from build123d import *

# Parameters (mm, degrees)
ESBO_O1_R           = 30
ESBO_O1_R_2         = 25
BOSS_EXTRUDE1_DEPTH = 1.57
BOSS_EXTRUDE2_START = -1.57
BOSS_EXTRUDE2_DEPTH = 1.57
BOSS_EXTRUDE3_DEPTH = 1.57
BOSS_EXTRUDE4_START = -1.57
SKETCH4_R           = 22.5
BOSS_EXTRUDE4_DEPTH = 1.57
BOSS_EXTRUDE5_START = -1.57
BOSS_EXTRUDE5_DEPTH = 1.57
CUT_EXTRUDE1_START  = -1.57
CUT_EXTRUDE1_DEPTH  = 1.57
CUT_EXTRUDE2_START  = -10
CUT_EXTRUDE2_DEPTH  = 10
EXTRUDE_THIN2_START = -1.57
EXTRUDE_THIN2_DEPTH = 1.57
BOSS_EXTRUDE9_DEPTH = 1.57


# Read off the part's stored shape, not the designer's step: Extrude-Thin2
with BuildPart() as part:
    # Esboço1 → Boss-Extrude1 (new body)
    with BuildSketch(Plane.XY):
        Circle(ESBO_O1_R)
        Circle(ESBO_O1_R_2, mode=Mode.SUBTRACT)
    extrude(amount=BOSS_EXTRUDE1_DEPTH)

    # Sketch1 → Boss-Extrude2 (add)
    with BuildSketch(Plane.XY.offset(1.57).offset(BOSS_EXTRUDE2_START)):
        with BuildLine():
            Line((-25.800536663, -15.307916512), (-15, -35))
            Line((-15, -35), (-15, -25.980762114))
            ThreePointArc((-15, -25.980762114), (-21.086686707, -21.338970071), (-25.800536663, -15.307916512))
        make_face()
        with BuildLine():
            Line((-15, -35), (0, -35))
            Line((0, -35), (0, -30))
            ThreePointArc((0, -30), (-7.764571353, -28.977774789), (-15, -25.980762114))
            Line((-15, -25.980762114), (-15, -35))
        make_face()
        with BuildLine():
            Line((0, -35), (15, -35))
            Line((15, -35), (15, -25.980762114))
            ThreePointArc((15, -25.980762114), (7.764571353, -28.977774789), (0, -30))
            Line((0, -30), (0, -35))
        make_face()
        with BuildLine():
            Line((15, -25.980762114), (15, -35))
            Line((15, -35), (25.800536663, -15.307916512))
            ThreePointArc((25.800536663, -15.307916512), (21.086686707, -21.338970071), (15, -25.980762114))
        make_face()
    extrude(amount=BOSS_EXTRUDE2_DEPTH)

    # Sketch2 → Boss-Extrude3 (add)
    with BuildSketch(Plane.XY):
        with BuildLine():
            Line((-2.5, -25), (-2.5, -22.360679775))
            ThreePointArc((-2.5, -22.360679775), (-5.0328099, -21.929907079), (-7.5, -21.213203436))
            Line((-7.5, -21.213203436), (-7.5, -25))
            Line((-7.5, -25), (-2.5, -25))
        make_face()
        with BuildLine():
            ThreePointArc((7.5, -21.213203436), (5.0328099, -21.929907079), (2.5, -22.360679775))
            Line((2.5, -22.360679775), (2.5, -25))
            Line((2.5, -25), (7.5, -25))
            Line((7.5, -25), (7.5, -21.213203436))
        make_face()
    extrude(amount=BOSS_EXTRUDE3_DEPTH)

    # Sketch4 → Boss-Extrude4 (add)
    with BuildSketch(Plane.XY.offset(1.57).offset(BOSS_EXTRUDE4_START)):
        Circle(SKETCH4_R)
    extrude(amount=BOSS_EXTRUDE4_DEPTH)

    # Sketch5 → Boss-Extrude5 (add)
    with BuildSketch(Plane.XY.offset(1.57).offset(BOSS_EXTRUDE5_START)):
        with BuildLine():
            Line((2.5, -24.874685928), (-2.5, -24.874685928))
            ThreePointArc((-2.5, -24.874685928), (0, -25), (2.5, -24.874685928))
        make_face()
    extrude(amount=BOSS_EXTRUDE5_DEPTH)

    # Sketch6 → Cut-Extrude1 (cut)
    with BuildSketch(Plane.XY.offset(1.57).offset(CUT_EXTRUDE1_START)):
        with BuildLine():
            Line((-2.5, -22.360679775), (2.5, -22.360679775))
            ThreePointArc((2.5, -22.360679775), (0, -22.5), (-2.5, -22.360679775))
        make_face()
    extrude(amount=CUT_EXTRUDE1_DEPTH, mode=Mode.SUBTRACT)

    # Sketch7 → Cut-Extrude2 (cut)
    with BuildSketch(Plane.XY.offset(1.57).offset(CUT_EXTRUDE2_START)):
        with BuildLine():
            add(Edge.make_bspline(
                [(-20.323456945, -14.558746437), (-13.043190103, -24.874685928), (-7.5, -24.874685928)],
                knots=[0, 0, 0, 1, 1, 1], degree=2))
            Line((-7.5, -24.874685928), (-7.5, -23.848480035))
            ThreePointArc((-7.5, -23.848480035), (-14.666662084, -20.245716172), (-20.323456945, -14.558746437))
        make_face()
        with BuildLine():
            add(Edge.make_bspline(
                [(20.323456945, -14.558746437), (13.043190103, -24.874685928), (7.5, -24.874685928)],
                knots=[0, 0, 0, 1, 1, 1], degree=2))
            ThreePointArc((20.323456945, -14.558746437), (14.666662084, -20.245716172), (7.5, -23.848480035))
            Line((7.5, -23.848480035), (7.5, -24.874685928))
        make_face()
    extrude(amount=CUT_EXTRUDE2_DEPTH, mode=Mode.SUBTRACT)

    # Extrude-Thin2 outline → Extrude-Thin2 (add)
    with BuildSketch(Plane.XY.offset(1.57).offset(EXTRUDE_THIN2_START)):
        with BuildLine():
            add(Edge.make_bspline(
                [(-7.5, -22.360679775), (-16.957974034, -18.314631092), (-20.809324876, -8.556985344)],
                knots=[0, 0, 0, 0.902799725, 0.902799725, 0.902799725], degree=2))
            Line((-7.5, -22.360679775), (-7.5, -21.213203436))
            ThreePointArc((-7.5, -21.213203436), (-15.504819665, -16.30492463), (-20.809324876, -8.556985344))
        make_face()
    extrude(amount=EXTRUDE_THIN2_DEPTH)

    # Sketch10 → Boss-Extrude9 (add)
    with BuildSketch(Plane.XY.offset(1.57)):
        with BuildLine():
            Line((2.499590074, -22.36028679), (2.499590074, -20.208780459))
            Line((2.499590074, -20.208780459), (21.573238209, -6.389263197))
            add(Edge.make_bspline(
                [(7.499590074, -22.36028679), (17.975860478, -17.878618737), (21.573238209, -6.389263197)],
                knots=[0, 0, 0, 1, 1, 1], degree=2))
            Line((7.499590074, -22.36028679), (2.499590074, -22.36028679))
        make_face()
    extrude(amount=-BOSS_EXTRUDE9_DEPTH)


solid = part.part
Read the model definition and answer for the solid it produces. Units are mm, in the model's axes. A direction names the side the tool comes from. Coordinates: 2 decimals unless noted, no trailing zeros. Loops run counter-clockwise (first coordinate to the right, second up) from the corner with the lowest first, then second, coordinate; pieces in that order, holes last. Notation, with made-up numbers: (70, 32) -> (80, 32) arc R35 ccw to (80, 71) -> close; hole circle Ø9 at (-24.75, -2). An arc over 180 degrees is marked (long way). Write item = value, one per line. Start each with the question number.
1) The part is cut by section A-A, the plane y = 0. Determine the outline of the cut face in (x, z).
2) The part is cut by section C-C, the plane x = 23.5. Determine the outline of the cut face in (y, z).
3) The part is cut by section B-B, the plane x = 0. Determine the outline of the cut face in (y, z), plus the area to 3 significant figures.
4) The part is cut by section D-D, the plane z = 1.05. State how many separate pieces and enclosed holes the cut face has, plus the area to 3 significant figures.
5) For faces 1 (the face through (2.5, -24, 1)), 2 (the face through (0, -2, 1.57)), determine the directions among +Z, -Z, +X, -X, +Y, -Y from which every point of the face is accessible in a straight line to the end or side of a thin tool.
6) Given P1, Ø0.5, axis at y = -24, z = 1, coming from the -X side, flat-ended and moving along its own axis, determine where the tip first touches the part or whether it passes through.
7) The mould has two halves that part along X. Classify faces 3 (the face through (0, -2, 0)), 4 (the face through (20.325, -25.292, 0.774)), 5 (the face through (7.5, -24, 1)): pulls with the +X half, pulls with the -X half, needs draft (parallel to the pull), parting line crosses it, or undercut.
8) Find the intervals of material crossed by L1, parallel to X at y = 0, z = 0.75; L2, parallel to Y at x = 0, z = 1.05; L3, parallel to X at y = 4.5, z = 0.55, in increasing order. Write a range as from..to.
Result:
q1.outline = (-30, 0) -> (-25, 0) -> (-25, 1.57) -> (-30, 1.57) -> close; (-22.5, 0) -> (22.5, 0) -> (22.5, 1.57) -> (-22.5, 1.57) -> close; (25, 0) -> (30, 0) -> (30, 1.57) -> (25, 1.57) -> close
q2.outline = (-19.5, 0) -> (-8.53, 0) -> (-8.53, 1.57) -> (-19.5, 1.57) -> close; (8.53, 0) -> (18.65, 0) -> (18.65, 1.57) -> (8.53, 1.57) -> close
q3.outline = (-35, 0) -> (-24.87, 0) -> (-24.87, 1.57) -> (-35, 1.57) -> close; (-22.36, 0) -> (22.5, 0) -> (22.5, 1.57) -> (-22.36, 1.57) -> close; (25, 0) -> (30, 0) -> (30, 1.57) -> (25, 1.57) -> close
q3.area = 94.2 mm²
q4.separate_pieces = 1
q4.enclosed_holes = 2
q4.area = 2,740 mm²
q5.face_1 = +Z, -Z
q5.face_2 = +Z, +X, -X, +Y, -Y
q6.P1 = -21.17
q7.face_3 = needs draft
q7.face_4 = pulls with the +X half
q7.face_5 = undercut
q8.L1 = -30..-25, -22.5..22.5, 25..30
q8.L2 = -35..-24.87, -22.36..22.5, 25..30
q8.L3 = -29.66..-24.59, -22.05..22.05, 24.59..29.66
